from build123d import *

# Parameters (mm, degrees)
BOSS_EXTRUDE1_DEPTH = 38.1
CUT_EXTRUDE2_REACH  = 122.881
SKETCH2_R           = 1.5
SKETCH2_R_2         = 5.5


with BuildPart() as part:
    # Sketch1 → Boss-Extrude1 (new body)
    with BuildSketch(Plane(origin=(0, 0, 0), x_dir=(0, 0, -1), z_dir=(1, 0, 0))):
        Polygon((-99.06, 57.86), (-99.06, 55.32), (0, 55.32), (0, 0), (-12.7, 0), (-12.7, -2.54), (15.24, -2.54), (15.24, 0), (2.54, 0), (2.54, 57.86), align=None)
    extrude(amount=BOSS_EXTRUDE1_DEPTH)

    # Sketch2 → Cut-Extrude2 (cut, up to next)
    with BuildSketch(Plane.XY, mode=Mode.PRIVATE) as cut_extrude2_sk1:
        with Locations((19.05, 26.42)):
            Circle(SKETCH2_R)
    cut_extrude2_tool1 = extrude(cut_extrude2_sk1.sketch, amount=-CUT_EXTRUDE2_REACH, mode=Mode.PRIVATE) & part.part
    # Sketch2 → Cut-Extrude2 (cut, up to next)
    with BuildSketch(Plane.XY, mode=Mode.PRIVATE) as cut_extrude2_sk2:
        with Locations((19.05, 9.42)):
            Circle(SKETCH2_R)
    cut_extrude2_tool2 = extrude(cut_extrude2_sk2.sketch, amount=-CUT_EXTRUDE2_REACH, mode=Mode.PRIVATE) & part.part
    # Sketch2 → Cut-Extrude2 (cut, up to next)
    with BuildSketch(Plane.XY, mode=Mode.PRIVATE) as cut_extrude2_sk3:
        with Locations((27.55, 17.92)):
            Circle(SKETCH2_R)
    cut_extrude2_tool3 = extrude(cut_extrude2_sk3.sketch, amount=-CUT_EXTRUDE2_REACH, mode=Mode.PRIVATE) & part.part
    # Sketch2 → Cut-Extrude2 (cut, up to next)
    with BuildSketch(Plane.XY, mode=Mode.PRIVATE) as cut_extrude2_sk4:
        with Locations((10.55, 17.92)):
            Circle(SKETCH2_R)
    cut_extrude2_tool4 = extrude(cut_extrude2_sk4.sketch, amount=-CUT_EXTRUDE2_REACH, mode=Mode.PRIVATE) & part.part
    # Sketch2 → Cut-Extrude2 (cut, up to next)
    with BuildSketch(Plane.XY, mode=Mode.PRIVATE) as cut_extrude2_sk5:
        with Locations((19.05, 17.92)):
            Circle(SKETCH2_R_2)
    cut_extrude2_tool5 = extrude(cut_extrude2_sk5.sketch, amount=-CUT_EXTRUDE2_REACH, mode=Mode.PRIVATE) & part.part
    add(cut_extrude2_tool1.solids().sort_by_distance((19.05, 26.42, 0))[0], mode=Mode.SUBTRACT)
    add(cut_extrude2_tool2.solids().sort_by_distance((19.05, 9.42, 0))[0], mode=Mode.SUBTRACT)
    add(cut_extrude2_tool3.solids().sort_by_distance((27.55, 17.92, 0))[0], mode=Mode.SUBTRACT)
    add(cut_extrude2_tool4.solids().sort_by_distance((10.55, 17.92, 0))[0], mode=Mode.SUBTRACT)
    add(cut_extrude2_tool5.solids().sort_by_distance((19.05, 17.92, 0))[0], mode=Mode.SUBTRACT)


solid = part.part
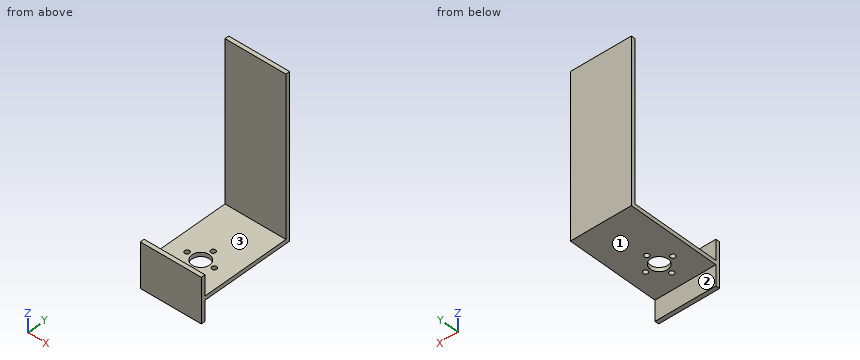
Source: CAD feature listing. Evaluate the final solid. Frame: model axes, mm. Face numbers are marked on the shaded views. Coordinates: 2 decimals unless noted, no trailing zeros. Loops run counter-clockwise (first coordinate to the right, second up) from the corner with the lowest first, then second, coordinate; pieces in that order, holes last. Notation, with made-up numbers: (-20.75, 24) -> (-2.75, 24) arc R19 ccw to (-2.75, 61) -> close; hole circle Ø4 at (17, 52.5). An arc over 180 degrees is marked (long way). Answer in a Markdown table with one row per item. Add a question column.
Q1. Section A-A on x = 27.55. Return the cut outline in (y, z), and give its area (3 significant figures).
Q2. Section C-C on x = 19.05. Return the cut outline in (y, z).
Q3. Ray query, line 1 along Y through (x, z) = (19.05, -1.85); line 2 along Y through (x, z) = (27.55, -1); line 3 along X through (y, z) = (17, -1). Return the intervals inside material, ascending.
Q4. Section D-D on z = 7. Return the cut outline in (x, y), and give its area (3 significant figures).
Q5. Section B-B on y = 17.92. Return the cut outline in (x, z).
Q6. Contact query for flat-ended pins moving along their axis: pin 1 Ø2.5 at (x, y) = (19.05, 9.42) entering from -Z; pin 2 Ø3 at (x, z) = (11.5, 32.5) entering from -Y; pin 3 Ø4 at (x, y) = (10.55, 17.92) entering from -Z; pin 4 Ø2 at (x, y) = (23.5, -1) entering from +Z. Output: stop coordinate, or through.
Q7. Pull-direction query (Y, two-part tool) for the marked faces 1, 2 and 3; classes: pulls with the +Y half, pulls with the -Y half, needs draft (parallel to the pull), parting line crosses it, or undercut.
Computed values:
| question | item | result |
|---|---|---|
| 1 | outline | (-2.54, -15.24) -> (0, -15.24) -> (0, -2.54) -> (16.42, -2.54) -> (16.42, 0) -> (0, 0) -> (0, 12.7) -> (-2.54, 12.7) -> close; (19.42, -2.54) -> (57.86, -2.54) -> (57.86, 99.06) -> (55.32, 99.06) -> (55.32, 0) -> (19.42, 0) -> close |
| 1 | area | 462 mm^2 |
| 2 | outline | (-2.54, -15.24) -> (0, -15.24) -> (0, -2.54) -> (7.92, -2.54) -> (7.92, 0) -> (0, 0) -> (0, 12.7) -> (-2.54, 12.7) -> close; (10.92, -2.54) -> (12.42, -2.54) -> (12.42, 0) -> (10.92, 0) -> close; (23.42, -2.54) -> (24.92, -2.54) -> (24.92, 0) -> (23.42, 0) -> close; (27.92, -2.54) -> (57.86, -2.54) -> (57.86, 99.06) -> (55.32, 99.06) -> (55.32, 0) -> (27.92, 0) -> close |
| 3 | line 1 | y = -2.54 to 7.92, 10.92 to 12.42, 23.42 to 24.92, 27.92 to 57.86 |
| 3 | line 2 | y = -2.54 to 16.42, 19.42 to 57.86 |
| 3 | line 3 | x = 0 to 9.37, 11.73 to 13.63, 24.47 to 26.37, 28.73 to 38.1 |
| 4 | outline | (0, -2.54) -> (38.1, -2.54) -> (38.1, 0) -> (0, 0) -> close; (0, 55.32) -> (38.1, 55.32) -> (38.1, 57.86) -> (0, 57.86) -> close |
| 4 | area | 194 mm^2 |
| 5 | outline | (0, -2.54) -> (9.05, -2.54) -> (9.05, 0) -> (0, 0) -> close; (12.05, -2.54) -> (13.55, -2.54) -> (13.55, 0) -> (12.05, 0) -> close; (24.55, -2.54) -> (26.05, -2.54) -> (26.05, 0) -> (24.55, 0) -> close; (29.05, -2.54) -> (38.1, -2.54) -> (38.1, 0) -> (29.05, 0) -> close |
| 6 | pin 1 | passes through |
| 6 | pin 2 | stops at y = 55.32 |
| 6 | pin 3 | stops at z = -2.54 |
| 6 | pin 4 | stops at z = 12.7 |
| 7 | face 1 | needs draft |
| 7 | face 2 | pulls with the +Y half |
| 7 | face 3 | undercut |
